from build123d import *

# Parameters (mm, degrees)
SKETCH1_R           = 46
SKETCH1_R_2         = 3
SKETCH1_R_3         = 1.4
BOSS_EXTRUDE1_DEPTH = 3
SKETCH5_R           = 1
CUT_EXTRUDE1_DEPTH  = 3
SKETCH6_R           = 1
CUT_EXTRUDE2_DEPTH  = 3


with BuildPart() as part:
    # Sketch1 → Boss-Extrude1 (new body)
    with BuildSketch(Plane(origin=(0, 0, 0), x_dir=(1, 0, 0), z_dir=(0, 1, 0))):
        Circle(SKETCH1_R)
        Circle(SKETCH1_R_2, mode=Mode.SUBTRACT)
        with Locations((0, 9.5)):
            Circle(SKETCH1_R_3, mode=Mode.SUBTRACT)
        with Locations((8.227241336, 4.75)):
            Circle(SKETCH1_R_3, mode=Mode.SUBTRACT)
        with Locations((8.227241336, -4.75)):
            Circle(SKETCH1_R_3, mode=Mode.SUBTRACT)
        with Locations((0, -9.5)):
            Circle(SKETCH1_R_3, mode=Mode.SUBTRACT)
        with Locations((-8.227241336, -4.75)):
            Circle(SKETCH1_R_3, mode=Mode.SUBTRACT)
        with Locations((-8.227241336, 4.75)):
            Circle(SKETCH1_R_3, mode=Mode.SUBTRACT)
    extrude(amount=BOSS_EXTRUDE1_DEPTH)

    # Sketch5 → Cut-Extrude1 (cut)
    with BuildSketch(Plane.XY.offset(46)):
        with Locations((0, 1.5)):
            Circle(SKETCH5_R)
    extrude(amount=-CUT_EXTRUDE1_DEPTH, mode=Mode.SUBTRACT)

    # Sketch6 → Cut-Extrude2 (cut)
    with BuildSketch(Plane.XY.offset(-46)):
        with Locations((0, 1.5)):
            Circle(SKETCH6_R)
    extrude(amount=CUT_EXTRUDE2_DEPTH, mode=Mode.SUBTRACT)


solid = part.part
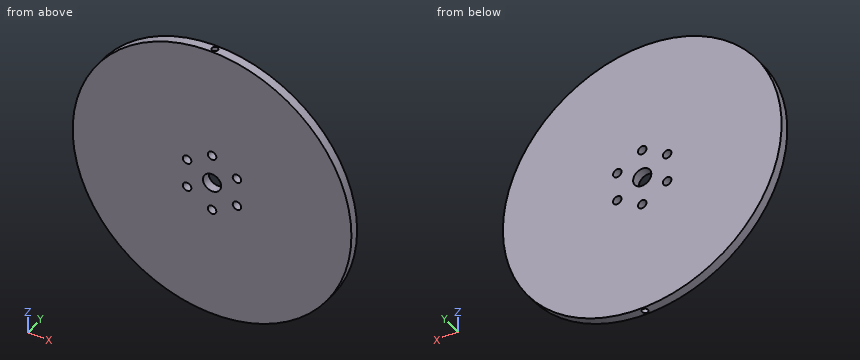
Could you check a few things on this model? Use its own coordinates, in mm. Give positions to 0.01 mm unless a question says otherwise; leave off trailing zeros. Order: outer loops, then holes, each group sorted by start corner. A loop starts at its lowest first (then second) coordinate and runs counter-clockwise, first axis right, second up. Notation, with made-up numbers: (68, -7) - (119, -7) arc R22 cw to (119, 26) - close; hole circle Ø5 at (53, -1). An arc over 180 degrees is marked (long way). One line per question, with ' | ' between items. Start each with the question number.
Item 1: I want a section at A-A on z = 0. Write out the boundary of the cut face in (x, y), then the cut area to 3 significant figures.
Item 2: I need wall thicknesses on probe 1 along X at (y, z) = (1.95, 0); probe 2 along Z at (x, y) = (0.5, 0.3); probe 3 along X at (y, z) = (2, -4.75). Which ranges of each line are inside material? Lowest first, please. Write a range as [from, to].
Item 3: I want a section at B-B on y = 1.5. Write out the boundary of the cut face in (x, z).
Item 4: I'm going to push flat-ended pins straight in: pin 1 Ø1.7 at (x, z) = (-8.23, 4.75) entering from -Y; pin 2 Ø1 at (y, z) = (1, -15) entering from +X; pin 3 Ø12 at (x, z) = (-9.5, 22.5) entering from -Y; pin 4 Ø1.8 at (x, y) = (0, 1.5) entering from -Z. Where does each tip first touch, or does it pass through?
Item 5: I want a section at C-C on z = -9.5. Write out the boundary of the cut face in (x, y), then the cut area to 3 significant figures.
Item 6: I want a section at D-D on x = -33. Write out the boundary of the cut face in (y, z), then the cut area to 3 significant figures.
Verdict:
1) outline: (-46, 0) - (-3, 0) - (-3, 3) - (-46, 3) - close; (3, 0) - (46, 0) - (46, 3) - (3, 3) - close | area: 258 mm^2
2) probe 1: [-46, -3], [3, 46] | probe 2: [-46, -10.81], [-8.19, -2.96], [2.96, 8.19], [10.81, 46] | probe 3: [-45.75, -9.63], [-6.83, 6.83], [9.63, 45.75]
3) outline: (-1, -45.99) - (-1, -43) - (1, -43) - (1, -45.99) arc R46 ccw to (1, 45.99) - (1, 43) - (-1, 43) - (-1, 45.99) arc R46 ccw to start; hole circle Ø2.8 at (-8.23, -4.75); hole circle Ø2.8 at (-8.23, 4.75); hole circle Ø6 at (0, 0); hole circle Ø2.8 at (0, -9.5); hole circle Ø2.8 at (0, 9.5); hole circle Ø2.8 at (8.23, -4.75); hole circle Ø2.8 at (8.23, 4.75)
4) pin 1: through | pin 2: x = 43.65 | pin 3: y = 0 | pin 4: z = -43
5) outline: (-45.01, 0) - (-1.4, 0) - (-1.4, 3) - (-45.01, 3) - close; (1.4, 0) - (45.01, 0) - (45.01, 3) - (1.4, 3) - close | area: 262 mm^2
6) outline: (0, -32.05) - (3, -32.05) - (3, 32.05) - (0, 32.05) - close | area: 192 mm^2
